```python
from build123d import *

# Parameters (mm, degrees)
F0_R          = 12.7
F1_DEPTH      = 25.4
F2_R          = 5.7092426067
F3_DEPTH      = 19.05
F5_R          = 12.7
F5_R_2        = 11.6839995608
F6_DEPTH      = 6.35
F6_DEPTH_BACK = 6.35
F7_DEPTH      = 3.175
F7_DEPTH_BACK = 3.175
F8_DEPTH      = 1.27
F8_DEPTH_BACK = 1.27
F9_SIZE       = 1.27


with BuildPart() as f1:
    # F0 (on Top) → F1 (new body)
    with BuildSketch(Plane.XY):
        Circle(F0_R)
    extrude(amount=F1_DEPTH)

    # F2 (on face) → F3 (cut)
    with BuildSketch(Plane.XY.offset(25.4)):
        Circle(F2_R)
    extrude(amount=-F3_DEPTH, mode=Mode.SUBTRACT)

    # F5 (on offset) → F6 (cut, two sides)
    with BuildSketch(Plane.XY.offset(12.7)) as f6_sk:
        Circle(F5_R)
        Circle(F5_R_2, mode=Mode.SUBTRACT)
    extrude(amount=-F6_DEPTH, mode=Mode.SUBTRACT)
    extrude(f6_sk.sketch, amount=F6_DEPTH_BACK, mode=Mode.SUBTRACT)

    # F5 (on offset) → F7 (join, two sides)
    with BuildSketch(Plane.XY.offset(12.7)) as f7_sk:
        Circle(F5_R)
        Circle(F5_R_2, mode=Mode.SUBTRACT)
    extrude(amount=F7_DEPTH)
    extrude(f7_sk.sketch, amount=-F7_DEPTH_BACK)

    # F5 (on offset) → F8 (cut, two sides)
    with BuildSketch(Plane.XY.offset(12.7)) as f8_sk:
        Circle(F5_R)
        Circle(F5_R_2, mode=Mode.SUBTRACT)
    extrude(amount=-F8_DEPTH, mode=Mode.SUBTRACT)
    extrude(f8_sk.sketch, amount=F8_DEPTH_BACK, mode=Mode.SUBTRACT)

    # F9
    f9_edges = [f1.edges().sort_by_distance(p)[0] for p in [
        (-12.7, 0, 0),
    ]]
    chamfer(f9_edges, length=F9_SIZE)


solid = f1.part
```
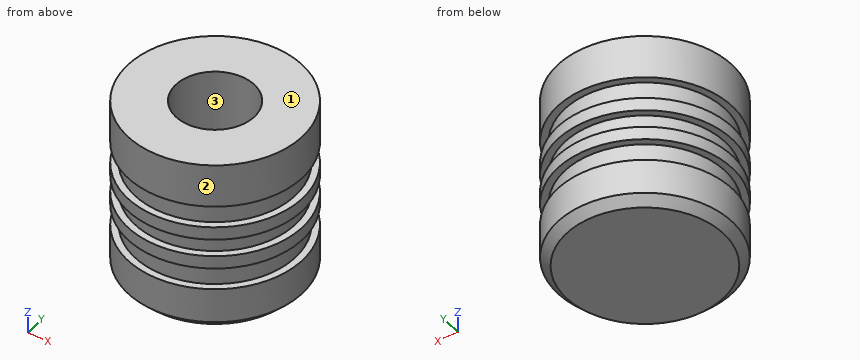
CAD build for the part. Positions are in the model's coordinates, mm. Face numbers are marked on the shaded views. Give positions to 0.01 mm unless a question says otherwise; leave off trailing zeros. Write each loop counter-clockwise with the first axis right and the second up, starting at its lowest first coordinate (ties: lowest second). Pieces come first, ordered by that corner, then holes. Notation, with made-up numbers: (-38.5, 36) -> (2.5, 36) arc R9 cw to (2.5, 46) -> close; hole circle Ø1 at (43, -21.75). An arc over 180 degrees is marked (long way). Write each question's results on one line, items separated by ' | '.
1. Two-plate mould, pull along X, no slides. Class the marked faces 1, 2 and 3: pulls with the +X half, pulls with the -X half, needs draft (parallel to the pull), parting line crosses it, or undercut.
Geometry check:
face 1: needs draft | face 2: parting line crosses it | face 3: undercut
2. Drop flat-ended pins along their axis: P1, Ø2, axis at x = -4.5, z = 22.5, coming from the -Y side; P2, Ø6, axis at x = -3.5, z = 22, coming from the +Y side; P3, Ø10, axis at y = -9, z = 7.5, coming from the -X side. Give the stop position or say it passes through.
Geometry check:
P1: y = -12.21 | P2: y = 12.69 | P3: x = -12.01
3. Cut at C-C, the plane z = 12.25. Write the cut outline in (x, y), then the cut area to 3 significant figures.
Geometry check:
outline: circle Ø23.37 at (0, 0); hole circle Ø11.42 at (0, 0) | area: 326 mm²
4. Wall check: probe 1 along Z at (x, y) = (-9.5, 7.5) (3 decimals); probe 2 along Z at (x, y) = (-5, 10.75) (3 decimals); probe 3 along X at (y, z) = (0.25, 24.25). Give the ranges that are in metal, low to high. Write a range as [from, to].
Geometry check:
probe 1: [0.674, 6.35], [9.525, 11.43], [13.97, 15.875], [19.05, 25.4] | probe 2: [0.426, 6.35], [9.525, 11.43], [13.97, 15.875], [19.05, 25.4] | probe 3: [-12.7, -5.7], [5.7, 12.7]
5. Cut at D-D, the plane z = 15.5. Write the cut outline in (x, y).
Geometry check:
outline: circle Ø25.4 at (0, 0); hole circle Ø11.42 at (0, 0)
